Design review of the part shown in the three views and the two pictorial views. Dimensions are in mm from the part's minimum x, y and z. A direction names the side the tool comes from. Coordinates: 2 decimals unless noted, no trailing zeros. Write each loop counter-clockwise with the first axis right and the second up, starting at its lowest first coordinate (ties: lowest second). Pieces come first, ordered by that corner, then holes. Notation, with made-up numbers: (-35.75, 67) - (23.25, 67) arc R13 cw to (23.25, 90) - close; hole circle Ø10 at (19.5, 69). An arc over 180 degrees is marked (long way). Write each question's results on one line, items separated by ' | '.
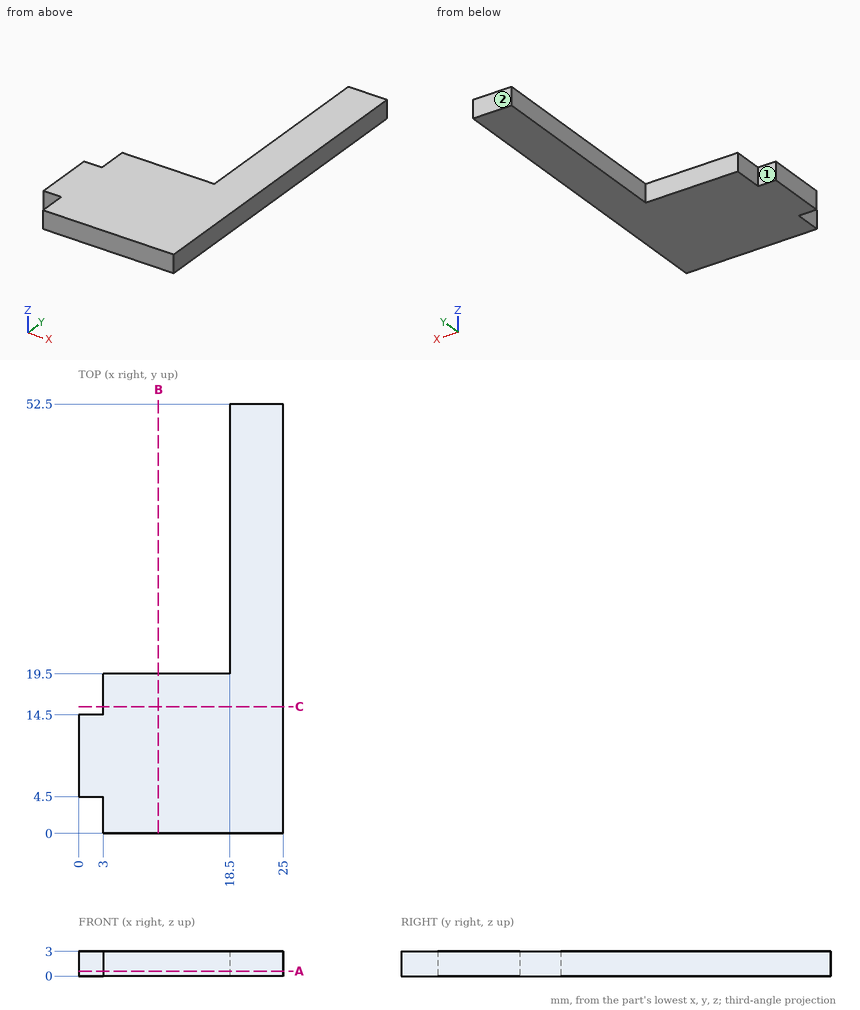
Q1. Take a section at A-A on z = 0.6. State the section outline as (x, y) points, plus the area to 4 significant figures.
Results found:
outline: (0, 4.5) - (3, 4.5) - (3, 0) - (25, 0) - (25, 52.5) - (18.5, 52.5) - (18.5, 19.5) - (3, 19.5) - (3, 14.5) - (0, 14.5) - close | area: 673.5 mm2
Q2. Take a section at C-C on y = 15.5. State the section outline as (x, z) points, plus the area to 3 significant figures.
Results found:
outline: (3, 0) - (25, 0) - (25, 3) - (3, 3) - close | area: 66.0 mm2
Q3. For pin 1 (12 mm diameter, centred on x = 16, y = 44.5, fed in from -Z); pin 2 (0.9 mm diameter, centred on y = 17.5, z = 1, fed in from -X); pin 3 (1 mm diameter, centred on y = 36.5, z = 1, fed in from -X); pin 4 (1 mm diameter, centred on x = 17.5, y = 41, fed in from +Z), all flat-tipped, find the tip position at first contact; note any pin that passes through.
Results found:
pin 1: z = 0 | pin 2: x = 3 | pin 3: x = 18.5 | pin 4: through
Q4. Take a section at B-B on x = 9.75. State the section outline as (y, z) points.
Results found:
outline: (0, 0) - (19.5, 0) - (19.5, 3) - (0, 3) - close
Q5. Wall thickness on line 1 along X through (y, z) = (44.5, 2.35); line 2 along Y through (x, z) = (18, 2.4); line 3 along X through (y, z) = (18, 2.4): over which ranges is each line inside the solid? List them lowest first. Write a range as from..to.
Results found:
line 1: 18.5..25 | line 2: 0..19.5 | line 3: 3..25
Q6. For the marked faces 1 and 2, list the 3-axis set-ups (+Z, -Z, +X, -X, +Y, -Y) from which the entire face can be reached by the end or side of a thin tool; tool diameter is ignored.
Results found:
face 1: +Z, -Z, -X, +Y | face 2: +Z, -Z, +X, -X, +Y
